from build123d import *
from build123d.topology import SkipClean

# Parameters (mm, degrees)
EXTRUDE_1_DEPTH          = 65
SHELL_1_T                = -3.5
CUT_EXTRUDE_3_DEPTH      = 86.293611
CUT_EXTRUDE_3_DEPTH_BACK = 86.293611
FILLET_1_R               = 15
SKETCH_3_W               = 40
SKETCH_3_H               = 3.5
CUT_EXTRUDE_4_DEPTH      = 61.5
SKETCH_4_R               = 5
CUT_EXTRUDE_5_DEPTH      = 96.865792
EXTRUDE_START            = 3
SKETCH_5_R               = 29
EXTRUDE_2_DEPTH          = 3
FILLET_2_R               = 3
SKETCH_6_R               = 8
CUT_EXTRUDE_6_DEPTH      = 83.657426


with BuildPart() as part:
    # 草图1 → 凸台-拉伸1 (new body)
    with BuildSketch(Plane.XY):
        with BuildLine():
            Line((-23.5, -16.992645), (-23.5, -47))
            Line((-23.5, -47), (23.5, -47))
            Line((23.5, -47), (23.5, -16.992645))
            ThreePointArc((23.5, -16.992645), (0, 29), (-23.5, -16.992645))
        make_face()
    extrude(amount=EXTRUDE_1_DEPTH)

    # 抽壳1
    shell_1_openings = [part.faces().sort_by_distance(p)[0] for p in [
        (0, -9.973122, 65),
    ]]
    offset(amount=SHELL_1_T, openings=shell_1_openings, kind=Kind.INTERSECTION)

    # 草图2 → 切除-拉伸3 (cut, two sides: drawn at the far end of the back side and taken through both)
    with BuildSketch(Plane(origin=(0, 0, 0), x_dir=(0, 0, -1), z_dir=(1, 0, 0)).offset(-CUT_EXTRUDE_3_DEPTH_BACK)):
        with BuildLine():
            Line((-5, 232.659495), (-5, 29))
            ThreePointArc((-5, 29), (-8.409806, 15.608871), (-17.808738, 5.479252))
            Line((-17.808738, 5.479252), (-65, -25))
            Line((-65, -25), (-236.079414, -135.494453))
            Line((-236.079414, -135.494453), (-581.070507, 81.046318))
            Line((-581.070507, 81.046318), (-349.991093, 449.200266))
            Line((-349.991093, 449.200266), (-5, 232.659495))
        make_face()
    extrude(amount=CUT_EXTRUDE_3_DEPTH + CUT_EXTRUDE_3_DEPTH_BACK, mode=Mode.SUBTRACT)

    # 圆角1
    fillet_1_edges = [part.edges().sort_by_distance(p)[0] for p in [
        (-23.5, -16.992645, 26.301076),
        (23.5, -16.992645, 26.301076),
    ]]
    fillet(fillet_1_edges, radius=FILLET_1_R)

    # 草图3 → 切除-拉伸4 (cut)
    with BuildSketch(Plane.XY.offset(65)):
        with Locations((0, -45.25)):
            Rectangle(SKETCH_3_W, SKETCH_3_H)
    extrude(amount=-CUT_EXTRUDE_4_DEPTH, mode=Mode.SUBTRACT)

    # 草图4 → 切除-拉伸5 (cut, through all)
    with BuildSketch(Plane(origin=(23.5, 0, 0), x_dir=(0, 0, -1), z_dir=(1, 0, 0))):
        with Locations(Location((-57, -34, 0), (0, 0, 90))):
            Circle(SKETCH_4_R)
    extrude(amount=-CUT_EXTRUDE_5_DEPTH, mode=Mode.SUBTRACT)

    # 草图5 → 凸台-拉伸2 (add)
    with SkipClean():  # the faces are left unmerged after this step: merging them gives an invalid solid
        with BuildSketch(Plane(origin=(0, 0, 0), x_dir=(-1, 0, 0), z_dir=(0, 0, -1)).offset(EXTRUDE_START)):
            Circle(SKETCH_5_R)
        extrude(amount=-EXTRUDE_2_DEPTH)

    # 圆角2
    fillet_2_edges = [part.edges().sort_by_distance(p)[0] for p in [
        (29, 0, -3),
    ]]
    fillet(fillet_2_edges, radius=FILLET_2_R - 0.0001)  # a hair under: the kernel refuses the full size

    # 草图6 → 切除-拉伸6 (cut, through all)
    with BuildSketch(Plane.XY.offset(3.5)):
        Circle(SKETCH_6_R)
    extrude(amount=-CUT_EXTRUDE_6_DEPTH, mode=Mode.SUBTRACT)


solid = part.part
The listing builds one solid part. Answer for the finished solid, in the listing's coordinates (mm). A direction names the side the tool comes from. Coordinates: 2 decimals unless noted, no trailing zeros. Order: outer loops, then holes, each group sorted by start corner. A loop starts at its lowest first (then second) coordinate and runs counter-clockwise, first axis right, second up. Notation, with made-up numbers: (42.25, -38.5) -> (96.25, -38.5) arc R12 cw to (96.25, -16.5) -> close; hole circle Ø4 at (41, 59). An arc over 180 degrees is marked (long way). Answer in a Markdown table with one row per item. Add a question column.
Item 1: Determine the mould class of faces 1 (the face through (23.99, -17.5, 30.05)), 2 (the face through (-23.963, -17.603, 30.052)), 3 (the face through (-5.41, 6.14, -3)), 4 (the face through (21.093, -14.329, 16.525)) for opening direction X: +X half, -X half, draft (parallel to the pull), parting line (faces both ways), or undercut.
Item 2: Which of the six approach directions +Z, -Z, +X, -X, +Y, -Y give full straight-line access (tool end or side, diameter ignored) to faces 5 (the face through (20, -32, 35)), 6 (the face through (23.5, -34, 32)), 7 (the face through (-23.5, -34, 32))?
Item 3: Find section C-C (z = 7.5). Write down the section's boundary in (x, y) (3 decimals).
Item 4: Find section D-D (y = 0). Write down the section's boundary in (x, z).
Item 5: Find section A-A (y = -34). Write down the section's boundary in (x, z), then the cut area to 3 significant figures.
Item 6: Each of these flat-tipped pins is pushed along its axis until it touches: P1, Ø13, axis at y = -30, z = 34.5, coming from the +X side; P2, Ø20.5, axis at y = -32, z = 31, coming from the -X side; P3, Ø15.5, axis at y = -26, z = 38, coming from the +X side. Where does it stop, or does it pass through?
Item 7: Find the intervals of material crossed by L1, parallel to Z at x = -22, y = -34; L2, parallel to Z at x = -13, y = -11.5; L3, parallel to X at y = -16, z = 14.5, in increasing order. Write a range as from..to.
Result set:
| question | item | result |
|---|---|---|
| 1 | face 1 | +X half |
| 1 | face 2 | -X half |
| 1 | face 3 | draft |
| 1 | face 4 | undercut |
| 2 | face 5 | +Z, -Y |
| 2 | face 6 | +Z, -Z, +X, -Y |
| 2 | face 7 | +Z, -Z, -X, -Y |
| 3 | outline | (-25.375, -14.04) arc R15 cw to (-23.5, -21.301) -> (-23.5, -47) -> (-20, -47) -> (-20, -15.819) arc R25.5 cw to (-18.608, 17.435) -> (-23.174, 17.435) arc R29 ccw to start; (18.608, 17.435) arc R25.5 cw to (20, -15.819) -> (20, -47) -> (23.5, -47) -> (23.5, -21.301) arc R15 cw to (25.375, -14.04) arc R29 ccw to (23.174, 17.435) -> close |
| 4 | outline | (-29, 0) arc R3 ccw to (-26, -3) -> (-8, -3) -> (-8, 3.5) -> (-25.5, 3.5) -> (-25.5, 26.29) -> (-29, 26.29) -> close; (8, -3) -> (26, -3) arc R3 ccw to (29, 0) -> (29, 26.29) -> (25.5, 26.29) -> (25.5, 3.5) -> (8, 3.5) -> close |
| 5 | outline | (-23.5, 0) -> (23.5, 0) -> (23.5, 52) -> (20, 52) -> (20, 3.5) -> (-20, 3.5) -> (-20, 52) -> (-23.5, 52) -> close; (-23.5, 62) -> (-20, 62) -> (-20, 65) -> (-23.5, 65) -> close; (20, 62) -> (23.5, 62) -> (23.5, 65) -> (20, 65) -> close |
| 5 | area | 525 mm² |
| 6 | P1 | stops at x = 23.5 |
| 6 | P2 | stops at x = -23.5 |
| 6 | P3 | stops at x = 23.81 |
| 7 | L1 | z = 0..52, 62..65 |
| 7 | L2 | z = -3..3.5 |
| 7 | L3 | x = -24.47..-20, 20..24.47 |
